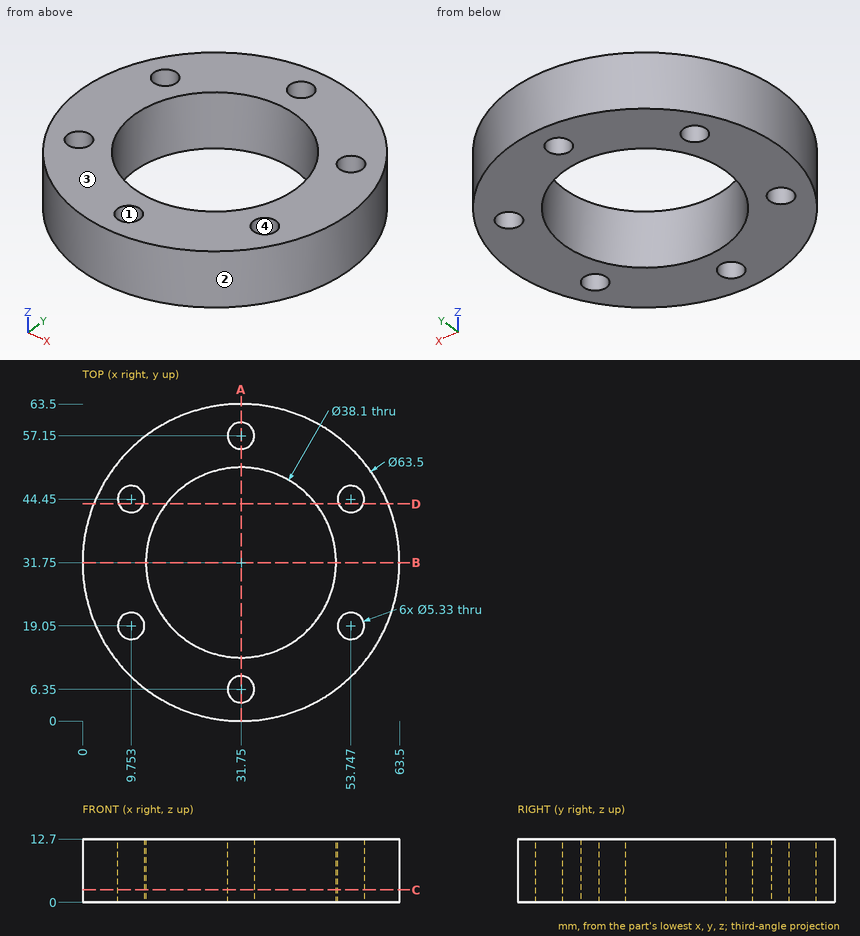
Here's the drawing with two shaded views (mm, measured from the low corner). I have some questions. Coordinates: 2 decimals unless noted, no trailing zeros. Write each loop counter-clockwise with the first axis right and the second up, starting at its lowest first coordinate (ties: lowest second). Pieces come first, ordered by that corner, then holes. Notation, with made-up numbers: (82, 61.5) -> (124, 61.5) arc R18 ccw to (124, 68.5) -> close; hole circle Ø10 at (-31.5, 51). An arc over 180 degrees is marked (long way). One line per question, with ' | ' between items. Start each with the question number.
1. Will these pins go through, and if not, where does the flat tip stop? P1, Ø2, axis at x = 33.5, z = 7.5, coming from the -Y side; P2, Ø1.5, axis at y = 7.5, z = 8, coming from the -X side; P3, Ø7, axis at x = 9.75, y = 44.45, coming from the -Z side; P4, Ø1.5, axis at x = 54, z = 3.5, coming from the -Y side.
2. If we section it at D-D (y = 43.5): Please give me the cut outline in (x, z).
3. If we section it at A-A (x = 31.75): Please give me the cut outline in (y, z) (3 decimals).
4. Thinking about a two-plate mould opening in Y: for the marked faces 1, 2, 3 and 4, which applies, pulls with the +Y half, pulls with the -Y half, needs draft (parallel to the pull), parting line crosses it, or undercut?
5. If we section it at C-C (z = 2.5): Please give me the cut outline in (x, y) (3 decimals).
6. Please list where these lines run through material, in increasing order: line 1 along Y through (x, z) = (31.75, 5.75) (3 decimals); line 2 along Y through (x, z) = (8.5, 8.5); line 3 along Y through (x, z) = (54, 1.25).
7. If we section it at B-B (y = 31.75): Please give me the cut outline in (x, z), and give its area (3 significant figures).
Return value:
1) P1: stops at y = 0.01 | P2: stops at x = 10.4 | P3: stops at z = 0 | P4: stops at y = 8.39
2) outline: (2.25, 0) -> (7.26, 0) -> (7.26, 12.7) -> (2.25, 12.7) -> close; (12.24, 0) -> (16.76, 0) -> (16.76, 12.7) -> (12.24, 12.7) -> close; (46.74, 0) -> (51.26, 0) -> (51.26, 12.7) -> (46.74, 12.7) -> close; (56.24, 0) -> (61.25, 0) -> (61.25, 12.7) -> (56.24, 12.7) -> close
3) outline: (0, 0) -> (3.685, 0) -> (3.685, 12.7) -> (0, 12.7) -> close; (9.015, 0) -> (12.7, 0) -> (12.7, 12.7) -> (9.015, 12.7) -> close; (50.8, 0) -> (54.485, 0) -> (54.485, 12.7) -> (50.8, 12.7) -> close; (59.815, 0) -> (63.5, 0) -> (63.5, 12.7) -> (59.815, 12.7) -> close
4) face 1: undercut | face 2: parting line crosses it | face 3: needs draft | face 4: undercut
5) outline: circle Ø63.5 at (31.75, 31.75); hole circle Ø5.33 at (9.753, 19.05); hole circle Ø5.33 at (9.753, 44.45); hole circle Ø38.1 at (31.75, 31.75); hole circle Ø5.33 at (31.75, 6.35); hole circle Ø5.33 at (31.75, 57.15); hole circle Ø5.33 at (53.747, 19.05); hole circle Ø5.33 at (53.747, 44.45)
6) line 1: y = 0 to 3.685, 9.015 to 12.7, 50.8 to 54.485, 59.815 to 63.5 | line 2: y = 10.13 to 16.7, 21.4 to 42.1, 46.8 to 53.37 | line 3: y = 9.1 to 16.4, 21.7 to 41.8, 47.1 to 54.4
7) outline: (0, 0) -> (12.7, 0) -> (12.7, 12.7) -> (0, 12.7) -> close; (50.8, 0) -> (63.5, 0) -> (63.5, 12.7) -> (50.8, 12.7) -> close | area: 323 mm²
